Geometry check sheet. Reference: the model listing, model coordinates, mm. Give positions to 0.01 mm unless a question says otherwise; leave off trailing zeros. Loops run counter-clockwise (first coordinate to the right, second up) from the corner with the lowest first, then second, coordinate; pieces in that order, holes last. Notation, with made-up numbers: (6.25, 79) -> (15.25, 79) arc R12 ccw to (15.25, 89) -> close; hole circle Ø1 at (79.5, 69). An arc over 180 degrees is marked (long way). One line per question, with ' | ' between items.
from build123d import *

# Parameters (mm, degrees)
F1_DEPTH     = 12.7
F2_SIZE2     = 6.35
F2_SIZE      = 2.54
F2_2_SIZE2   = 6.34999
F2_2_SIZE    = 2.53999
F3_T1_DEPTH  = 121.4602589597
F3_T3_DEPTH  = 121.4603587348
F3_T5_DEPTH  = 2.54
F3_T7_DEPTH  = 2.6322967076
F3_S11_W     = 5.08
F3_S11_H     = 5.08
F3_T12_DEPTH = 5.08
F3_S17_W     = 5.08
F3_S17_H     = 5.08
F3_T18_DEPTH = 5.08
F3_S23_W     = 5.08
F3_S23_H     = 5.08
F3_T24_DEPTH = 5.08
F3_S29_W     = 5.08
F3_S29_H     = 5.08
F3_T30_DEPTH = 5.08


# Not quite as in the source:
# - a fillet or chamfer that OpenCascade refuses, or shapes differently, is made with other operations: its cross-section is extruded or revolved along the edge and cut away or added
# - a fillet or chamfer is up to 0.001 mm smaller than in the source, because OpenCascade refuses the exact size


with BuildPart() as f1:
    # F0 (on Top) → F1 (new body)
    with BuildSketch(Plane.XY):
        Polygon((75.9397223592, -6.3961483538), (75.9397223592, 6.3961483538), (-12.4434158206, 6.3961483538), (-75.9397223592, 0), (-12.4434158206, -6.3961483538), align=None)
    extrude(amount=F1_DEPTH)

    # F2
    f2_edges = [f1.edges().sort_by_distance(p)[0] for p in [
        (-44.191569, -3.198074, 12.7),
        (-44.191569, 3.198074, 12.7),
    ]]
    f2_side = f1.faces().sort_by_distance((14.475683, 0, 12.7))[0]
    chamfer(f2_edges, length=F2_SIZE, length2=F2_SIZE2, reference=f2_side)

    # F2#2 (size 2.54 and 6.35 in the source; OpenCascade refuses exactly that, so slightly less here)
    f2_2_edges = [f1.edges().sort_by_distance(p)[0] for p in [
        (-44.191569, -3.198074, 0),
        (-44.191569, 3.198074, 0),
    ]]
    f2_2_side = f1.faces().sort_by_distance((14.475683, 0, 0))[0]
    chamfer(f2_2_edges, length=F2_2_SIZE, length2=F2_2_SIZE2, reference=f2_2_side)

    # F3: fillet of radius 5.08 on 8 edges, made by hand

    # F3_s2 → F3_t1 (cut)
    with BuildSketch(Plane.YZ.offset(-50.6005366005)):
        with BuildLine():
            ThreePointArc((-6.3961483538, 7.62), (-4.9082508022, 11.2121024484), (-1.3161483538, 12.7))
            Line((-1.3161483538, 12.7), (-6.3961483538, 12.7))
            Line((-6.3961483538, 12.7), (-6.3961483538, 7.62))
        make_face()
        with BuildLine():
            ThreePointArc((1.3161483538, 12.7), (4.9082508022, 11.2121024484), (6.3961483538, 7.62))
            Line((6.3961483538, 7.62), (6.3961483538, 12.7))
            Line((6.3961483538, 12.7), (1.3161483538, 12.7))
        make_face()
    extrude(amount=F3_T1_DEPTH, mode=Mode.SUBTRACT)

    # F3_s4 → F3_t3 (cut)
    with BuildSketch(Plane.YZ.offset(-50.6006363756)):
        with BuildLine():
            ThreePointArc((-6.3961483538, 5.08), (-4.9082508022, 1.4878975516), (-1.3161483538, 0))
            Line((-1.3161483538, 0), (-6.3961483538, 0))
            Line((-6.3961483538, 0), (-6.3961483538, 5.08))
        make_face()
        with BuildLine():
            ThreePointArc((1.3161483538, 0), (4.9082508022, 1.4878975516), (6.3961483538, 5.08))
            Line((6.3961483538, 5.08), (6.3961483538, 0))
            Line((6.3961483538, 0), (1.3161483538, 0))
        make_face()
    extrude(amount=F3_T3_DEPTH, mode=Mode.SUBTRACT)

    # F3_s6 → F3_t5 (cut)
    with BuildSketch(Plane.XY.offset(5.08)):
        with BuildLine():
            ThreePointArc((70.8597223592, -6.3961483538), (74.4518248076, -4.9082508022), (75.9397223592, -1.3161483538))
            Line((75.9397223592, -1.3161483538), (75.9397223592, -6.3961483538))
            Line((75.9397223592, -6.3961483538), (70.8597223592, -6.3961483538))
        make_face()
        with BuildLine():
            ThreePointArc((75.9397223592, 1.3161483538), (74.4518248076, 4.9082508022), (70.8597223592, 6.3961483538))
            Line((70.8597223592, 6.3961483538), (75.9397223592, 6.3961483538))
            Line((75.9397223592, 6.3961483538), (75.9397223592, 1.3161483538))
        make_face()
    extrude(amount=F3_T5_DEPTH, mode=Mode.SUBTRACT)

    # F3_s8 → F3_t7 (cut)
    with BuildSketch(Plane.XZ.offset(-1.3161483538)):
        with BuildLine():
            ThreePointArc((70.8597223592, 12.7), (74.4518248076, 11.2121024484), (75.9397223592, 7.62))
            Line((75.9397223592, 7.62), (75.9397223592, 12.7))
            Line((75.9397223592, 12.7), (70.8597223592, 12.7))
        make_face()
        with BuildLine():
            ThreePointArc((70.8597223592, 0), (74.4518248076, 1.4878975516), (75.9397223592, 5.08))
            Line((75.9397223592, 5.08), (75.9397223592, 0))
            Line((75.9397223592, 0), (70.8597223592, 0))
        make_face()
    extrude(amount=F3_T7_DEPTH, mode=Mode.SUBTRACT)


with BuildPart() as f3_tool10:
    # F3_s11 → F3_t12 (new body)
    with BuildSketch(Plane.XZ.offset(1.3161483538)):
        with Locations((73.3997223592, 10.16)):
            Rectangle(F3_S11_W, F3_S11_H)
    extrude(amount=F3_T12_DEPTH)

    # F3_s13 → F3_t14 (revolve, cut)
    with BuildSketch(Plane(origin=(70.8597223592, -1.3161483538, 7.62), x_dir=(-0.7071067812, 0, -0.7071067812), z_dir=(-0.7071067812, 0, 0.7071067812))):
        with BuildLine():
            ThreePointArc((0, -5.08), (5.08, 0), (0, 5.08))
            Line((0, 5.08), (0, -5.08))
        make_face()
    revolve(axis=Axis((70.8597223592, -1.3161483538, 7.62), (0, -1, 0)), mode=Mode.SUBTRACT)


with BuildPart() as f1_1:
    add(f1.part)

    # F3_t9: cut F3_tool10
    add(f3_tool10.part, mode=Mode.SUBTRACT)


with BuildPart() as f3_tool16:
    # F3_s17 → F3_t18 (new body)
    with BuildSketch(Plane.XZ.offset(1.3161483538)):
        with Locations((73.3997223592, 2.54)):
            Rectangle(F3_S17_W, F3_S17_H)
    extrude(amount=F3_T18_DEPTH)

    # F3_s19 → F3_t20 (revolve, cut)
    with BuildSketch(Plane(origin=(70.8597223592, -1.3161483538, 5.08), x_dir=(-0.7071067812, 0, 0.7071067812), z_dir=(0.7071067812, 0, 0.7071067812))):
        with BuildLine():
            ThreePointArc((0, -5.08), (5.08, 0), (0, 5.08))
            Line((0, 5.08), (0, -5.08))
        make_face()
    revolve(axis=Axis((70.8597223592, -1.3161483538, 5.08), (0, -1, 0)), mode=Mode.SUBTRACT)


with BuildPart() as f1_2:
    add(f1_1.part)

    # F3_t15: cut F3_tool16
    add(f3_tool16.part, mode=Mode.SUBTRACT)


with BuildPart() as f3_tool22:
    # F3_s23 → F3_t24 (new body)
    with BuildSketch(Plane.XZ.offset(-1.3161483538)):
        with Locations((73.3997223592, 2.54)):
            Rectangle(F3_S23_W, F3_S23_H)
    extrude(amount=-F3_T24_DEPTH)

    # F3_s25 → F3_t26 (revolve, cut)
    with BuildSketch(Plane(origin=(70.8597223592, 1.3161483538, 5.08), x_dir=(-0.7071067812, 0, 0.7071067812), z_dir=(-0.7071067812, 0, -0.7071067812))):
        with BuildLine():
            ThreePointArc((0, -5.08), (5.08, 0), (0, 5.08))
            Line((0, 5.08), (0, -5.08))
        make_face()
    revolve(axis=Axis((70.8597223592, 1.3161483538, 5.08), (0, 1, 0)), mode=Mode.SUBTRACT)


with BuildPart() as f1_3:
    add(f1_2.part)

    # F3_t21: cut F3_tool22
    add(f3_tool22.part, mode=Mode.SUBTRACT)


with BuildPart() as f3_tool28:
    # F3_s29 → F3_t30 (new body)
    with BuildSketch(Plane.XZ.offset(-1.3161483538)):
        with Locations((73.3997223592, 10.16)):
            Rectangle(F3_S29_W, F3_S29_H)
    extrude(amount=-F3_T30_DEPTH)

    # F3_s31 → F3_t32 (revolve, cut)
    with BuildSketch(Plane(origin=(70.8597223592, 1.3161483538, 7.62), x_dir=(-0.7071067812, 0, -0.7071067812), z_dir=(0.7071067812, 0, -0.7071067812))):
        with BuildLine():
            ThreePointArc((0, -5.08), (5.08, 0), (0, 5.08))
            Line((0, 5.08), (0, -5.08))
        make_face()
    revolve(axis=Axis((70.8597223592, 1.3161483538, 7.62), (0, 1, 0)), mode=Mode.SUBTRACT)


with BuildPart() as f1_4:
    add(f1_3.part)

    # F3_t27: cut F3_tool28
    add(f3_tool28.part, mode=Mode.SUBTRACT)


solid = f1_4.part
Item 1: Scan lines: probe 1 along Z at (x, y) = (4, 1.75); probe 2 along Z at (x, y) = (24.5, -3.75); probe 3 along Y at (x, z) = (-35, 8.75). Record each from-to range of solid material in increasing order.
Result:
probe 1: 0.02 to 12.68 | probe 2: 0.62 to 12.08 | probe 3: -3.16 to 3.16
Item 2: Sectioned sample at A-A (x = 29.5). Record the cut outline in (y, z), plus the area to 3 significant figures.
Result:
outline: (-6.4, 5.08) arc R5.08 ccw to (-1.32, 0) -> (1.32, 0) arc R5.08 ccw to (6.4, 5.08) -> (6.4, 7.62) arc R5.08 ccw to (1.32, 12.7) -> (-1.32, 12.7) arc R5.08 ccw to (-6.4, 7.62) -> close | area: 140 mm2
Item 3: Sectioned sample at B-B (z = 3.25). Record the cut outline in (x, y), plus the area to 3 significant figures.
Result:
outline: (-63.57, 0) -> (-3.46, -6.06) -> (70.86, -6.06) arc R4.74 ccw to (75.6, -1.32) -> (75.6, 1.32) arc R4.74 ccw to (70.86, 6.06) -> (-3.46, 6.06) -> close | area: 1,310 mm2
Item 4: Sectioned sample at D-D (z = 9.5). Record the cut outline in (x, y), plus the area to 3 significant figures.
Result:
outline: (-63.37, 0) -> (-3.45, -6.04) -> (70.86, -6.04) arc R4.72 ccw to (75.58, -1.32) -> (75.58, 1.32) arc R4.72 ccw to (70.86, 6.04) -> (-3.45, 6.04) -> close | area: 1,310 mm2
Item 5: Depth check by flat-ended pin: pin 1 Ø3 at (x, y) = (42, -3) entering from +Z; pin 2 Ø4 at (x, z) = (47, 1.5) entering from -Y; pin 3 Ø1.5 at (x, z) = (41.5, 2) entering from -Y. Enter the tip coordinate at first touch or a pass-through.
Result:
pin 1: z = 12.7 | pin 2: y = -6.14 | pin 3: y = -5.83
